Geometry check sheet. Reference: drawing and pictorial views, mm from the part's lowest x, y, z. A direction names the side the tool comes from. Round coordinates to 2 decimals unless told otherwise and drop trailing zeros. Write each loop counter-clockwise with the first axis right and the second up, starting at its lowest first coordinate (ties: lowest second). Pieces come first, ordered by that corner, then holes.
Item 1: Depth check by flat-ended pin: pin 1 (1.2 mm diameter, centred on x = 2, z = 6, fed in from -Y); pin 2 (2.5 mm diameter, centred on x = 4, z = 11.5, fed in from +Y); pin 3 (0.6 mm diameter, centred on x = 12, z = 12, fed in from -Y). Enter the tip coordinate at first touch or a pass-through.
Item 2: Section check A-A, the plane z = 11.5. Record the cut outline in (x, y).
Item 3: Set-up check for the marked faces 1 and 2: record each of +Z, -Z, +X, -X, +Y, -Y from which the full face is reachable in a straight line by a thin tool's end or side.
Item 4: Material ranges on line 1 along Z through (x, y) = (4, 50.8); line 2 along X through (y, z) = (12, 9); line 3 along Y through (x, z) = (10.25, 2.75), recorded low to high.
Item 5: Release check for a two-part mould opening along Z. For the marked faces 3, 4, 5 and 6 record: pulls with the +Z half, pulls with the -Z half, needs draft (parallel to the pull), parting line crosses it, or undercut.
Item 6: Section check B-B, the plane y = 36.5. Record the cut outline in (x, z), plus the area to 3 significant figures.
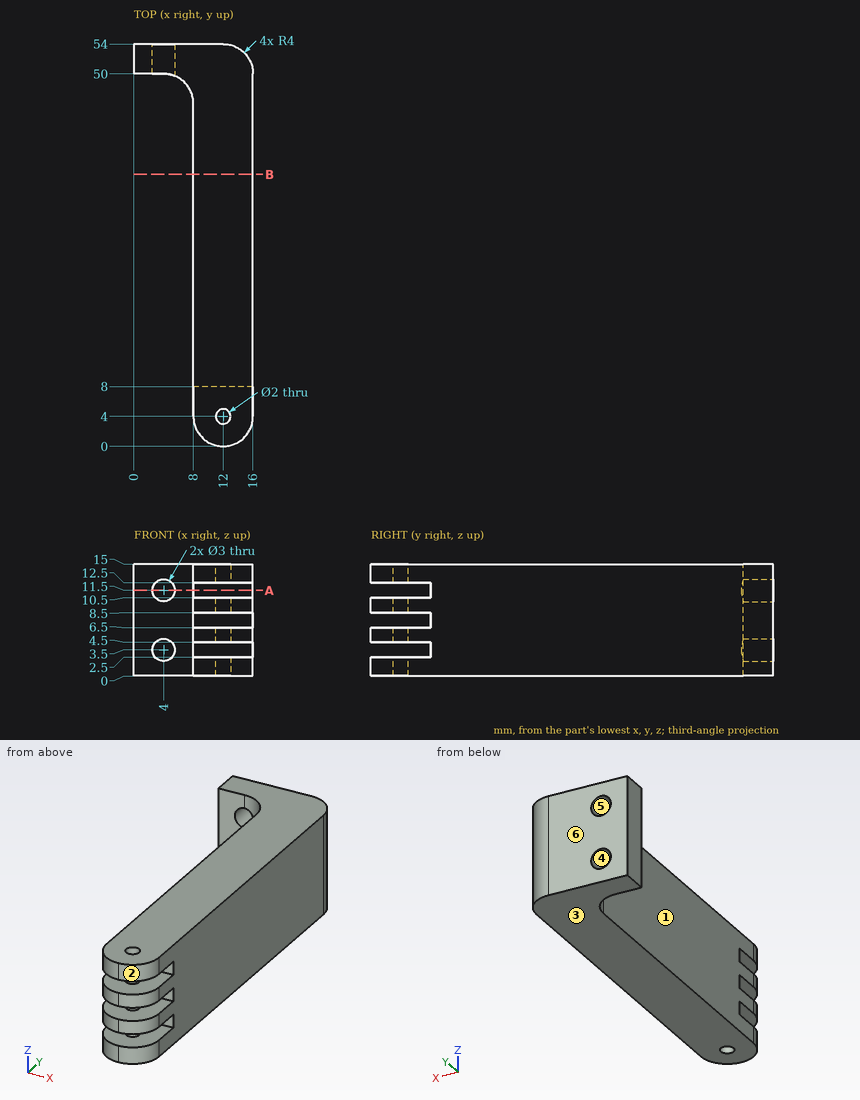
Values found:
1. pin 1: stops at y = 50
1. pin 2: passes through
1. pin 3: stops at y = 8
2. outline: (0, 50) - (2.5, 50) - (2.5, 54) - (0, 54) - close; (5.5, 49.71) arc R4 cw to (8, 46) - (8, 8) - (16, 8) - (16, 50) arc R4 ccw to (12, 54) - (5.5, 54) - close
3. face 1: +Z, -Z, -X, -Y
3. face 2: +Z, -Z, +X, -Y
4. line 1: z = 0 to 2, 5 to 10, 13 to 15
4. line 2: x = 8 to 16
4. line 3: y = 8 to 54
5. face 3: pulls with the -Z half
5. face 4: undercut
5. face 5: undercut
5. face 6: needs draft
6. outline: (8, 0) - (16, 0) - (16, 15) - (8, 15) - close
6. area: 120 mm2
